Here's how the part is built. I have some questions about the finished solid (model axes, mm). Face numbers are marked on the shaded views. A direction names the side the tool comes from. Round coordinates to 2 decimals unless told otherwise and drop trailing zeros. Write each loop counter-clockwise with the first axis right and the second up, starting at its lowest first coordinate (ties: lowest second). Pieces come first, ordered by that corner, then holes. Notation, with made-up numbers: (-8.75, 18) - (30.25, 18) arc R15 cw to (30.25, 30) - close; hole circle Ø2 at (-31, 15). An arc over 180 degrees is marked (long way). Use one line per item in the form item = value. Start each with the question number.
1. If I drill on line 1 along Z through (x, y) = (1, 8); line 2 along X through (y, z) = (-1.5, 26.5); line 3 along X through (y, z) = (0, 31), over which ranges is the centre line in solid material (lowest first)?
2. I want a section at B-B, the plane z = 35. List the corners of the cut face in (x, y) for me, plus the area to 3 significant figures.
3. I want a section at D-D, the plane x = -44. List the corners of the cut face in (y, z) for me (3 decimals).
4. Will these pins go through, and if not, where does the flat tip stop? pin 1 (3 mm diameter, centred on x = -121.5, z = 20.5, fed in from +Y); pin 2 (3 mm diameter, centred on y = 2, z = 34, fed in from +X); pin 3 (3 mm diameter, centred on y = -3, z = 19, fed in from +X); pin 4 (1 mm diameter, centred on x = 37.5, z = 13.5, fed in from -Y).
5. I want a section at C-C, the plane y = -8. List the corners of the cut face in (x, z) for me (3 decimals), plus the area to 3 significant figures.
6. Which directions (+Z, -Z, +X, -X, +Y, -Y) give clear straight access to the entire face, cutting with the end or side of a thin tool? Please do the marked faces 4 and 5.
7. We'd pull the mould along X, two halves only. Please class the marked faces 1, 2 and 3: +X half, -X half, draft (parallel to the pull), parting line (faces both ways), or undercut.
8. I want a section at A-A, the plane x = 26. List the corners of the cut face in (y, z) for me.
```python
from build123d import *

# Parameters (mm, degrees)
SKETCH1_R               = 6.35
SKETCH1_R_2             = 7.220009846
BOSS_EXTRUDE1_DEPTH     = 38.1
SKETCH2_W               = 50.8
SKETCH2_H               = 25.4
CUT_EXTRUDE1_DEPTH      = 6.35
CUT_EXTRUDE2_DEPTH      = 131.862598214
CUT_EXTRUDE2_DEPTH_BACK = 131.862598214
SKETCH5_W               = 76.2
SKETCH5_H               = 12.7
SKETCH4_W               = 76.2
SKETCH4_H               = 6.35
CUT_EXTRUDE3_DEPTH      = 31.75
SKETCH7_W               = 32.699691946
SKETCH7_H               = 6.35
CUT_EXTRUDE4_DEPTH      = 19.05


with BuildPart() as part:
    # Sketch1 → Boss-Extrude1 (new body)
    with BuildSketch(Plane.XY):
        with BuildLine():
            Line((-104.416317992, 20.723849372), (47.983682008, 20.723849372))
            ThreePointArc((47.983682008, 20.723849372), (67.033682008, 1.673849372), (47.983682008, -17.376150628))
            Line((47.983682008, -17.376150628), (-104.416317992, -17.376150628))
            ThreePointArc((-104.416317992, -17.376150628), (-123.466317992, 1.673849372), (-104.416317992, 20.723849372))
        make_face()
        with Locations(Location((47.983682008, 1.673849372, 0), (0, 0, 180))):
            Circle(SKETCH1_R, mode=Mode.SUBTRACT)
        with Locations(Location((-104.416317992, 1.673849372, 0), (0, 0, 180))):
            Circle(SKETCH1_R_2, mode=Mode.SUBTRACT)
    extrude(amount=BOSS_EXTRUDE1_DEPTH)

    # Sketch2 → Cut-Extrude1 (cut)
    with BuildSketch(Plane.XY.offset(38.1)):
        with Locations((-91.716317992, 1.673849372)):
            Rectangle(SKETCH2_W, SKETCH2_H)
    extrude(amount=-CUT_EXTRUDE1_DEPTH, mode=Mode.SUBTRACT)

    # Sketch5 → Cut-Extrude2 (cut, two sides: drawn at the far end of the back side and taken through both)
    with BuildSketch(Plane(origin=(0, 0, 0), x_dir=(1, 0, 0), z_dir=(0, 1, 0)).offset(-CUT_EXTRUDE2_DEPTH_BACK)):
        with Locations((35.283682008, -19.05)):
            Rectangle(SKETCH5_W, SKETCH5_H)
    extrude(amount=CUT_EXTRUDE2_DEPTH + CUT_EXTRUDE2_DEPTH_BACK, mode=Mode.SUBTRACT)

    # Sketch4 → Cut-Extrude3 (cut)
    with BuildSketch(Plane(origin=(0, 20.723849372, 0), x_dir=(1, 0, 0), z_dir=(0, 1, 0))):
        with Locations((-79.016317992, -19.05)):
            Rectangle(SKETCH4_W, SKETCH4_H)
    extrude(amount=-CUT_EXTRUDE3_DEPTH, mode=Mode.SUBTRACT)

    # Sketch7 → Cut-Extrude4 (cut)
    with BuildSketch(Plane(origin=(0, 20.723849372, 0), x_dir=(1, 0, 0), z_dir=(0, 1, 0))):
        with Locations((-118.381657109, -19.05)):
            Rectangle(SKETCH7_W, SKETCH7_H)
    extrude(amount=-CUT_EXTRUDE4_DEPTH, mode=Mode.SUBTRACT)


solid = part.part
```
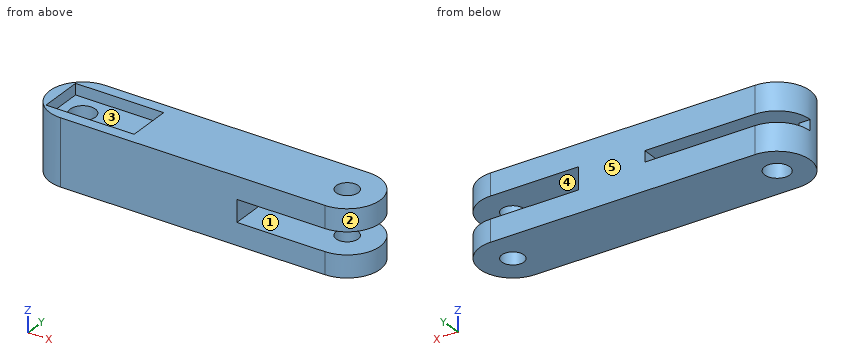
Model answer:
q1.line_1 = 0 to 12.7, 25.4 to 38.1
q1.line_2 = -123.2 to -110.9, -97.93 to 42.48, 53.48 to 66.77
q1.line_3 = -123.39 to -111.44, -97.39 to 41.86, 54.11 to 66.96
q2.outline = (-104.42, -17.38) - (47.98, -17.38) arc R19.05 ccw to (47.98, 20.72) - (-104.42, 20.72) arc R19.05 ccw to start; hole (-117.12, -11.03) - (-66.32, -11.03) - (-66.32, 14.37) - (-117.12, 14.37) - close; hole circle Ø12.7 at (47.98, 1.67)
q2.area = 5,530 mm2
q3.outline = (-17.376, 0) - (20.724, 0) - (20.724, 15.875) - (-11.026, 15.875) - (-11.026, 22.225) - (20.724, 22.225) - (20.724, 38.1) - (-17.376, 38.1) - close
q4.pin_1 = 1.67
q4.pin_2 = 67.03
q4.pin_3 = -2.82
q4.pin_4 = through
q5.outline = (-120.827, 0) - (64.395, 0) - (64.395, 12.7) - (-2.816, 12.7) - (-2.816, 25.4) - (64.395, 25.4) - (64.395, 38.1) - (-66.316, 38.1) - (-66.316, 31.75) - (-117.116, 31.75) - (-117.116, 38.1) - (-120.827, 38.1) - close; hole (-117.116, 15.875) - (-40.916, 15.875) - (-40.916, 22.225) - (-117.116, 22.225) - close
q5.area = 5,400 mm2
q6.face_4 = +X, +Y, -Y
q6.face_5 = +Z, -Z, +X, -X, +Y
q7.face_1 = draft
q7.face_2 = +X half
q7.face_3 = undercut
q8.outline = (-17.38, 0) - (20.72, 0) - (20.72, 12.7) - (-17.38, 12.7) - close; (-17.38, 25.4) - (20.72, 25.4) - (20.72, 38.1) - (-17.38, 38.1) - close
